Check sheet for the modelled part. Datum: model origin and axes. Units: mm. A direction names the side the tool comes from. Round coordinates to 2 decimals unless told otherwise and drop trailing zeros. Loops run counter-clockwise (first coordinate to the right, second up) from the corner with the lowest first, then second, coordinate; pieces in that order, holes last. Notation, with made-up numbers: (29.25, 84.5) - (35.25, 84.5) arc R32 cw to (35.25, 120.5) - close; hole circle Ø6 at (79, -12). An arc over 180 degrees is marked (long way). Put each result on its own line as item: value.
```python
from build123d import *

# Parameters (mm, degrees)
SKETCH_1_W      = 10
SKETCH_1_H      = 3
EXTRUDE_1_DEPTH = 3


with BuildPart() as part:
    # 草圖1 → 填料-伸長1 (new body)
    with BuildSketch(Plane.XY):
        Polygon((29.080711207, 23.718072979), (38.080711207, 23.718072979), (38.080711207, 37.718072979), (-61.919288793, 37.718072979), (-61.919288793, 23.718072979), (-52.919288793, 23.718072979), (-52.919288793, 26.718072979), (-42.919288793, 26.718072979), (-42.919288793, 23.718072979), (-28.919288793, 23.718072979), (-28.919288793, 26.718072979), (-18.919288793, 26.718072979), (-18.919288793, 23.718072979), (-4.919288793, 23.718072979), (-4.919288793, 26.718072979), (5.080711207, 26.718072979), (5.080711207, 23.718072979), (19.080711207, 23.718072979), (19.080711207, 26.718072979), (29.080711207, 26.718072979), align=None)
        with Locations((-47.919288793, 25.218072979)):
            Rectangle(SKETCH_1_W, SKETCH_1_H)
        with Locations((-23.919288793, 25.218072979)):
            Rectangle(SKETCH_1_W, SKETCH_1_H)
        with Locations((0.080711207, 25.218072979)):
            Rectangle(SKETCH_1_W, SKETCH_1_H)
        with Locations((24.080711207, 25.218072979)):
            Rectangle(SKETCH_1_W, SKETCH_1_H)
        Polygon((-52.919288793, 23.718072979), (-61.919288793, 23.718072979), (-61.919288793, 16.218072979), (-58.919288793, 16.218072979), (-58.919288793, 6.218072979), (-61.919288793, 6.218072979), (-61.919288793, -3.781927021), (-58.919288793, -3.781927021), (-58.919288793, -13.781927021), (-61.919288793, -13.781927021), (-61.919288793, -23.781927021), (-58.919288793, -23.781927021), (-58.919288793, -33.781927021), (-61.919288793, -33.781927021), (-61.919288793, -41.281927021), (-52.919288793, -41.281927021), (-52.919288793, -44.281927021), (-42.919288793, -44.281927021), (-42.919288793, -41.281927021), (-28.919288793, -41.281927021), (-28.919288793, -44.281927021), (-18.919288793, -44.281927021), (-18.919288793, -41.281927021), (-4.919288793, -41.281927021), (-4.919288793, -44.281927021), (5.080711207, -44.281927021), (5.080711207, -41.281927021), (19.080711207, -41.281927021), (19.080711207, -44.281927021), (29.080711207, -44.281927021), (29.080711207, -41.281927021), (38.080711207, -41.281927021), (38.080711207, -33.781927021), (35.080711207, -33.781927021), (35.080711207, -23.781927021), (38.080711207, -23.781927021), (38.080711207, -13.781927021), (35.080711207, -13.781927021), (35.080711207, -3.781927021), (38.080711207, -3.781927021), (38.080711207, 6.218072979), (35.080711207, 6.218072979), (35.080711207, 16.218072979), (38.080711207, 16.218072979), (38.080711207, 23.718072979), (29.080711207, 23.718072979), (19.080711207, 23.718072979), (5.080711207, 23.718072979), (-4.919288793, 23.718072979), (-18.919288793, 23.718072979), (-28.919288793, 23.718072979), (-42.919288793, 23.718072979), align=None)
    extrude(amount=EXTRUDE_1_DEPTH)


solid = part.part
```
Item 1: Section check B-B on y = 13. Enter the section's corners in (x, z).
Filled sheet:
outline: (-58.92, 0) - (35.08, 0) - (35.08, 3) - (-58.92, 3) - close
Item 2: Release check for a two-part mould opening along Y. For faces 1 (the flat face through (-57, -41.282, 1)), 2 (the flat face through (-60, 6.218, 1)), 3 (the flat face through (38.081, -19, 1)) record: +Y half, -Y half, draft (parallel to the pull), parting line (faces both ways), or undercut.
Filled sheet:
face 1: -Y half
face 2: undercut
face 3: draft
Item 3: Go/stop test with flat-tipped pins: pin 1 (1 mm diameter, centred on y = 9.5, z = 2, fed in from -X); pin 2 (1 mm diameter, centred on x = 7, z = 1.5, fed in from -Y); pin 3 (0.9 mm diameter, centred on y = -42, z = 1, fed in from -X). Record where each tip stops, or that it passes through.
Filled sheet:
pin 1: x = -58.92
pin 2: y = -41.28
pin 3: x = -52.92
Item 4: Tool access check on faces 4 (the flat face through (19.081, -43, 1)), 5 (the flat face through (-52.919, -43, 1)), 6 (the flat face through (-58.919, 11, 1)), 7 (the flat face through (29.081, -43, 1)). Record the directions out of +Z, -Z, +X, -X, +Y, -Y that give a thin tool (end or side, any length) a straight path to the whole face; none if there is none.
Filled sheet:
face 4: +Z, -Z, -Y
face 5: +Z, -Z, -X, -Y
face 6: +Z, -Z, -X
face 7: +Z, -Z, +X, -Y
Item 5: Thickness scan on line 1 (Y direction, x = 33.5, z = 1.25); line 2 (X direction, y = -13, z = 0.85). Record the ranges inside material, lowest first. Write a range as from..to.
Filled sheet:
line 1: -41.28..37.72
line 2: -58.92..35.08
Item 6: Section check A-A on x = -11. Enter the section's corners in (y, z), then the cut area to 3 significant figures.
Filled sheet:
outline: (-41.28, 0) - (37.72, 0) - (37.72, 3) - (-41.28, 3) - close
area: 237 mm²
